The model under review builds one solid part; all positions refer to its coordinate system, in mm. A direction names the side the tool comes from. Coordinates: 2 decimals unless noted, no trailing zeros. Order: outer loops, then holes, each group sorted by start corner. A loop starts at its lowest first (then second) coordinate and runs counter-clockwise, first axis right, second up. Notation, with made-up numbers: (-12.5, 24) -> (10.5, 24) arc R10 cw to (10.5, 41) -> close; hole circle Ø8 at (-28.5, 64.25). An arc over 180 degrees is marked (long way). Use one line per item in the form item = value.
from build123d import *

# Parameters (mm, degrees)
SKETCH_1_W           = 96.5
SKETCH_1_H           = 35
EXTRUDE_1_DEPTH      = 5.2
CUT_EXTRUDE_6_DEPTH  = 1.6
CUT_EXTRUDE_7_DEPTH  = 2.6
CUT_EXTRUDE_15_DEPTH = 5
SKETCH_7_W           = 8
SKETCH_7_H           = 17
CUT_EXTRUDE_16_DEPTH = 103.736994311
SKETCH_8_W           = 18.1
SKETCH_8_H           = 16.1
CUT_EXTRUDE_17_DEPTH = 1.66
CUT_EXTRUDE_18_REACH = 104.712
SKETCH_9_W           = 15.2
SKETCH_9_H           = 16.1
CHAMFER_1_SIZE       = 0.6
SKETCH_10_W          = 12.5
SKETCH_10_H          = 12.7
CUT_EXTRUDE_19_DEPTH = 1.66
CHAMFER_2_SIZE       = 0.8
CUT_EXTRUDE_20_DEPTH = 103.782732013
CHAMFER_4_SIZE       = 1
SKETCH_14_W          = 54.3
SKETCH_14_H          = 2
EXTRUDE_2_DEPTH      = 5.2
CHAMFER_5_SIZE       = 1
CUT_EXTRUDE_21_DEPTH = 1.66
CHAMFER_3_SIZE       = 1.5
CHAMFER_6_SIZE       = 1.6
SKETCH_16_W          = 2.1
SKETCH_16_H          = 6
CUT_EXTRUDE_22_DEPTH = 104.480867797
CUT_EXTRUDE_24_DEPTH = 104.480867797
CHAMFER_11_SIZE      = 2
CHAMFER_10_SIZE      = 0.4
CUT_EXTRUDE_START    = -4.2
SKETCH_21_W          = 6.7
SKETCH_21_H          = 9.8
CUT_EXTRUDE_26_DEPTH = 4.2
CHAMFER_9_SIZE       = 1.7
SKETCH_22_W          = 16
SKETCH_22_H          = 4
CUT_EXTRUDE_27_DEPTH = 4.2
CHAMFER_12_SIZE      = 2
SKETCH_24_R          = 1.5
CUT_EXTRUDE_28_DEPTH = 104.480867797
SKETCH_25_R          = 0.85
CUT_EXTRUDE_29_DEPTH = 3
SKETCH_26_R          = 0.85
CUT_EXTRUDE_30_DEPTH = 4
SKETCH_27_W          = 20
SKETCH_27_H          = 16.1
CUT_EXTRUDE_31_DEPTH = 104.480867797
SKETCH_28_W          = 10
SKETCH_28_H          = 1.4
EXTRUDE_3_DEPTH      = 4
CHAMFER_13_SIZE      = 2
CHAMFER_14_SIZE      = 2


# Some blends are built 0.0001 mm under size
with BuildPart() as part:
    # 草图1 → 凸台-拉伸1 (new body)
    with BuildSketch(Plane(origin=(0, 0, 0), x_dir=(1, 0, 0), z_dir=(0, 1, 0))):
        with Locations((48.25, 17.5)):
            Rectangle(SKETCH_1_W, SKETCH_1_H)
    extrude(amount=EXTRUDE_1_DEPTH)

    # 草图4 → 切除-拉伸6 (cut)
    with BuildSketch(Plane(origin=(0, 5.2, 0), x_dir=(1, 0, 0), z_dir=(0, 1, 0))):
        Polygon((1.8, 6.4), (49.9, 6.4), (49.9, 9.8), (57.9, 9.8), (57.9, 28.6), (49.9, 28.6), (49.9, 32), (1.8, 32), align=None)
    extrude(amount=-CUT_EXTRUDE_6_DEPTH, mode=Mode.SUBTRACT)

    # 草图5 → 切除-拉伸7 (cut)
    with BuildSketch(Plane(origin=(0, 3.6, 0), x_dir=(1, 0, 0), z_dir=(0, 1, 0))):
        Polygon((49.9, 9), (1.8, 9), (1.8, 32), (9.9, 32), (9.9, 29.4), (16.9, 29.4), (16.9, 24), (26.9, 24), (26.9, 32), (49.9, 32), (49.9, 28.6), (57.9, 28.6), (57.9, 9.8), (49.9, 9.8), align=None)
    extrude(amount=-CUT_EXTRUDE_7_DEPTH, mode=Mode.SUBTRACT)

    # 草图6 → 切除-拉伸15 (cut, symmetric)
    with BuildSketch(Plane(origin=(0, 1, 0), x_dir=(1, 0, 0), z_dir=(0, 1, 0))):
        Polygon((3.8, 32), (8.8, 32), (8.8, 9), (1.8, 9), (1.8, 21.5), (1, 21.5), (1, 32), align=None)
    extrude(amount=CUT_EXTRUDE_15_DEPTH, both=True, mode=Mode.SUBTRACT)

    # 草图7 → 切除-拉伸16 (cut, through all)
    with BuildSketch(Plane(origin=(0, 1, 0), x_dir=(1, 0, 0), z_dir=(0, 1, 0))):
        with Locations((43.879, 19.2)):
            Rectangle(SKETCH_7_W, SKETCH_7_H)
    extrude(amount=-CUT_EXTRUDE_16_DEPTH, mode=Mode.SUBTRACT)

    # 草图8 → 切除-拉伸17 (cut)
    with BuildSketch(Plane(origin=(0, 5.2, 0), x_dir=(1, 0, 0), z_dir=(0, 1, 0))):
        with Locations((79.45, 14.45)):
            Rectangle(SKETCH_8_W, SKETCH_8_H)
    extrude(amount=-CUT_EXTRUDE_17_DEPTH, mode=Mode.SUBTRACT)

    # 草图9 → 切除-拉伸18 (cut, up to next)
    with BuildSketch(Plane(origin=(0, 3.54, 0), x_dir=(1, 0, 0), z_dir=(0, 1, 0)), mode=Mode.PRIVATE) as cut_extrude_18_sk1:
        with Locations((79.2, 14.45)):
            Rectangle(SKETCH_9_W, SKETCH_9_H)
    cut_extrude_18_tool1 = extrude(cut_extrude_18_sk1.sketch, amount=-CUT_EXTRUDE_18_REACH, mode=Mode.PRIVATE) & part.part
    add(cut_extrude_18_tool1.solids().sort_by_distance((79.2, 3.54, -14.45))[0], mode=Mode.SUBTRACT)

    # 倒角1
    chamfer_1_edges = [part.edges().sort_by_distance(p)[0] for p in [
        (47.879, 1, -19.2),
    ]]
    chamfer(chamfer_1_edges, length=CHAMFER_1_SIZE)

    # 草图10 → 切除-拉伸19 (cut)
    with BuildSketch(Plane(origin=(0, 5.2, 0), x_dir=(1, 0, 0), z_dir=(0, 1, 0))):
        with Locations((64.15, 16.15)):
            Rectangle(SKETCH_10_W, SKETCH_10_H)
    extrude(amount=-CUT_EXTRUDE_19_DEPTH, mode=Mode.SUBTRACT)

    # 倒角2
    chamfer_2_edges = [part.edges().sort_by_distance(p)[0] for p in [
        (49.9, 3.1, -28.6),
        (49.9, 3.1, -9.8),
    ]]
    chamfer(chamfer_2_edges, length=CHAMFER_2_SIZE)

    # 草图12 → 切除-拉伸20 (cut, through all)
    with BuildSketch(Plane(origin=(0, 5.2, 0), x_dir=(1, 0, 0), z_dir=(0, 1, 0))):
        Polygon((96.5, 35), (77.5, 35), (77.5, 24), (90.5, 24), (90.5, 16), (96.5, 16), align=None)
    extrude(amount=-CUT_EXTRUDE_20_DEPTH, mode=Mode.SUBTRACT)

    # 倒角4
    chamfer_4_edges = [part.edges().sort_by_distance(p)[0] for p in [
        (96.5, 2.6, -16),
    ]]
    chamfer(chamfer_4_edges, length=CHAMFER_4_SIZE)

    # 草图14 → 凸台-拉伸2 (add)
    with BuildSketch(Plane(origin=(0, 5.2, 0), x_dir=(1, 0, 0), z_dir=(0, 1, 0))):
        with Locations((48.25, 36)):
            Rectangle(SKETCH_14_W, SKETCH_14_H)
    extrude(amount=-EXTRUDE_2_DEPTH)

    # 倒角5
    chamfer_5_edges = [part.edges().sort_by_distance(p)[0] for p in [
        (21.1, 2.6, -37),
        (75.4, 2.6, -37),
    ]]
    chamfer(chamfer_5_edges, length=CHAMFER_5_SIZE)

    # 草图15 → 切除-拉伸21 (cut)
    with BuildSketch(Plane(origin=(0, 5.2, 0), x_dir=(1, 0, 0), z_dir=(0, 1, 0))):
        Polygon((77.5, 32), (57.9, 32), (57.9, 30.602488817), (57.9, 22.5), (67.9, 22.5), (67.9, 27), (77.5, 27), align=None)
    extrude(amount=-CUT_EXTRUDE_21_DEPTH, mode=Mode.SUBTRACT)

    # 倒角3
    chamfer_3_edges = [part.edges().sort_by_distance(p)[0] for p in [
        (77.5, 3.54, -29.5),
    ]]
    chamfer(chamfer_3_edges, length=CHAMFER_3_SIZE)

    # 倒角6
    chamfer_6_edges = [part.edges().sort_by_distance(p)[0] for p in [
        (1.8, 4.4, -6.4),
    ]]
    chamfer(chamfer_6_edges, length=CHAMFER_6_SIZE)

    # 草图16 → 切除-拉伸22 (cut, through all)
    with BuildSketch(Plane(origin=(0, 5.2, 0), x_dir=(1, 0, 0), z_dir=(0, 1, 0))):
        with Locations((1.05, 3)):
            Rectangle(SKETCH_16_W, SKETCH_16_H)
        with Locations((95.45, 3)):
            Rectangle(SKETCH_16_W, SKETCH_16_H)
    extrude(amount=-CUT_EXTRUDE_22_DEPTH, mode=Mode.SUBTRACT)

    # 草图19 → 切除-拉伸24 (cut, through all)
    with BuildSketch(Plane(origin=(0, 5.2, 0), x_dir=(1, 0, 0), z_dir=(0, 1, 0))):
        Polygon((15, 0), (19.2, 0), (19.2, 2), (21.2, 2), (21.2, 4.2), (13, 4.2), (13, 2), (15, 2), align=None)
        Polygon((77.3, 2), (77.3, 0), (81.5, 0), (81.5, 2), (83.5, 2), (83.5, 4.2), (75.3, 4.2), (75.3, 2), align=None)
    extrude(amount=-CUT_EXTRUDE_24_DEPTH, mode=Mode.SUBTRACT)

    # 倒角11
    chamfer_11_edges = [part.edges().sort_by_distance(p)[0] for p in [
        (83.5, 2.6, -2),
        (75.3, 2.6, -2),
        (21.2, 2.6, -2),
        (13, 2.6, -2),
    ]]
    chamfer(chamfer_11_edges, length=CHAMFER_11_SIZE - 0.0001)  # a hair under: the kernel refuses the full size

    # 倒角10
    chamfer_10_edges = [part.edges().sort_by_distance(p)[0] for p in [
        (19.2, 2.6, 0),
        (15, 2.6, 0),
        (81.5, 2.6, 0),
        (77.3, 2.6, 0),
    ]]
    chamfer(chamfer_10_edges, length=CHAMFER_10_SIZE)

    # 草图21 → 切除-拉伸26 (cut)
    with BuildSketch(Plane(origin=(0, 5.2, 0), x_dir=(1, 0, 0), z_dir=(0, 1, 0)).offset(CUT_EXTRUDE_START)):
        with Locations((56.25, 4.9)):
            Rectangle(SKETCH_21_W, SKETCH_21_H)
    extrude(amount=CUT_EXTRUDE_26_DEPTH, mode=Mode.SUBTRACT)

    # 倒角9
    chamfer_9_edges = [part.edges().sort_by_distance(p)[0] for p in [
        (57.9, 3.54, -19.2),
        (58.75, 3.54, -9.8),
    ]]
    chamfer(chamfer_9_edges, length=CHAMFER_9_SIZE - 0.0001)  # a hair under: the kernel refuses the full size

    # 草图22 → 切除-拉伸27 (cut)
    with BuildSketch(Plane(origin=(0, 5.2, 0), x_dir=(1, 0, 0), z_dir=(0, 1, 0))):
        with Locations((44.9, 2)):
            Rectangle(SKETCH_22_W, SKETCH_22_H)
    extrude(amount=-CUT_EXTRUDE_27_DEPTH, mode=Mode.SUBTRACT)

    # 倒角12
    chamfer_12_edges = [part.edges().sort_by_distance(p)[0] for p in [
        (52.9, 3.1, -4),
    ]]
    chamfer(chamfer_12_edges, length=CHAMFER_12_SIZE)

    # 草图24 → 切除-拉伸28 (cut, through all)
    with BuildSketch(Plane(origin=(0, 5.2, 0), x_dir=(1, 0, 0), z_dir=(0, 1, 0))):
        with Locations(Location((30, 3, 0), (0, 0, 270))):
            Circle(SKETCH_24_R)
        with Locations(Location((66.5, 3, 0), (0, 0, 270))):
            Circle(SKETCH_24_R)
    extrude(amount=-CUT_EXTRUDE_28_DEPTH, mode=Mode.SUBTRACT)

    # 草图25 → 切除-拉伸29 (cut)
    with BuildSketch(Plane(origin=(0, 0, -35), x_dir=(-1, 0, 0), z_dir=(0, 0, -1))):
        with Locations((-10.2, 2.6)):
            Circle(SKETCH_25_R)
    extrude(amount=-CUT_EXTRUDE_29_DEPTH, mode=Mode.SUBTRACT)

    # 草图26 → 切除-拉伸30 (cut)
    with BuildSketch(Plane.XY):
        with Locations((86.25, 3)):
            Circle(SKETCH_26_R)
    extrude(amount=-CUT_EXTRUDE_30_DEPTH, mode=Mode.SUBTRACT)

    # 草图27 → 切除-拉伸31 (cut, through all)
    with BuildSketch(Plane(origin=(0, 5.2, 0), x_dir=(1, 0, 0), z_dir=(0, 1, 0))):
        with Locations((78.5, 14.45)):
            Rectangle(SKETCH_27_W, SKETCH_27_H)
    extrude(amount=-CUT_EXTRUDE_31_DEPTH, mode=Mode.SUBTRACT)

    # 草图28 → 凸台-拉伸3 (add)
    with BuildSketch(Plane.XZ):
        with Locations((81.5, -7.1)):
            Rectangle(SKETCH_28_W, SKETCH_28_H)
        with Locations((81.5, -21.8)):
            Rectangle(SKETCH_28_W, SKETCH_28_H)
    extrude(amount=-EXTRUDE_3_DEPTH)

    # 倒角13
    chamfer_13_edges = [part.edges().sort_by_distance(p)[0] for p in [
        (68.5, 4.37, -9.8),
    ]]
    chamfer(chamfer_13_edges, length=CHAMFER_13_SIZE)

    # 倒角14
    # the kernel refuses this chamfer: 2 mm, written as the material it takes off along each edge
    with BuildSketch(Plane(origin=(68.5, 3.54, -22.5), x_dir=(-0.9996219169112968, 0.027495876610586414, 0), z_dir=(0, 0, 1))) as chamfer_14_piece_1_section:
        Polygon((CHAMFER_14_SIZE * 0.999621916911, CHAMFER_14_SIZE * 0.0274958766106), (-CHAMFER_14_SIZE * 0.0274958766106, CHAMFER_14_SIZE * 0.999621916911), (0, 0), align=None)
    chamfer_14_piece_1 = extrude(amount=19.843365976, mode=Mode.PRIVATE)
    chamfer_14_piece_1 = split(chamfer_14_piece_1, bisect_by=Plane(origin=(63.791666667, 3.073333333, -12.508333333), z_dir=(0.7071067811865476, 0, -0.7071067811865476)), keep=Keep.TOP, mode=Mode.PRIVATE)
    add(chamfer_14_piece_1, mode=Mode.SUBTRACT)


solid = part.part
Item 1: We need section B-B (z = -31). Write out the cut boundary in (x, y).
Results found:
outline = (0, 0) -> (1, 0) -> (1, 5.2) -> (0, 5.2) -> close; (8.8, 0) -> (77.5, 0) -> (77.5, 2.04) -> (76, 3.54) -> (57.9, 3.54) -> (57.9, 5.2) -> (49.9, 5.2) -> (49.9, 1) -> (26.9, 1) -> (26.9, 3.6) -> (9.9, 3.6) -> (9.9, 1) -> (8.8, 1) -> close
Item 2: We need section C-C (z = -3). Write out the cut boundary in (x, y), plus the area to 3 significant figures.
Results found:
outline = (2.1, 0) -> (14, 0) -> (14, 5.2) -> (2.1, 5.2) -> close; (20.2, 0) -> (28.5, 0) -> (28.5, 5.2) -> (20.2, 5.2) -> close; (31.5, 0) -> (65, 0) -> (65, 5.2) -> (59.6, 5.2) -> (59.6, 1) -> (36.9, 1) -> (36.9, 5.2) -> (31.5, 5.2) -> close; (68, 0) -> (76.3, 0) -> (76.3, 5.2) -> (68, 5.2) -> close; (82.5, 0) -> (94.4, 0) -> (94.4, 5.2) -> (82.5, 5.2) -> close; hole circle Ø1.7 at (86.25, 3)
area = 287 mm²
Item 3: Tool access review of faces 4 (the face through (10, 1, -35)), 5 (the face through (26, 3.6, -8)), 6 (the face through (1, 3, -27)), 7 (the face through (36.9, 3, -2)): name each direction out of +Z, -Z, +X, -X, +Y, -Y from which nothing blocks a thin tool from reaching the whole face with its end or side.
Results found:
face_4 = -Z, -X, +Y, -Y
face_5 = +Y
face_6 = +Y, -Y
face_7 = +Z, +Y
Item 4: Draft analysis for pull direction Y (two halves, no side actions). For faces 1 (the face through (87.035, 2.674, -1.972)), 2 (the face through (26.9, 2, -28)), 3 (the face through (67.49, 2.55, -15.25)), state which applies: released by +Y, released by -Y, zero draft, split by the parting line, or undercut.
Results found:
face_1 = undercut
face_2 = zero draft
face_3 = released by +Y
Item 5: We need section D-D (x = 30). Write out the cut boundary in (y, z).
Results found:
outline = (0, -37) -> (5.2, -37) -> (5.2, -32) -> (1, -32) -> (1, -9) -> (3.6, -9) -> (3.6, -6.4) -> (5.2, -6.4) -> (5.2, -4.5) -> (0, -4.5) -> close; (0, -1.5) -> (5.2, -1.5) -> (5.2, 0) -> (0, 0) -> close
Item 6: We need section A-A (x = 47). Write out the cut boundary in (y, z).
Results found:
outline = (0, -37) -> (5.2, -37) -> (5.2, -32) -> (1, -32) -> (1, -27.7) -> (0, -27.7) -> close; (0, -10.7) -> (1, -10.7) -> (1, -9) -> (3.6, -9) -> (3.6, -6.4) -> (5.2, -6.4) -> (5.2, -4) -> (1, -4) -> (1, 0) -> (0, 0) -> close
Item 7: To check wall thickness, follow L1, parallel to X at y = 1.75, z = -28.5; L2, parallel to X at y = 0.35, z = -24.5; L3, parallel to Z at x = 87.5, y = 3.4. State the ranges of each line that lie inside material, in increasing order. Write a range as from..to.
Results found:
L1 = 0..1, 16.9..26.9, 57.9..77.5
L2 = 0..1, 8.8..39.88, 47.88..77.5
L3 = -24..-22.5, -6.4..0
Item 8: Clearance check with flat-ended pins moving along their axes: pin 1 (0.5 mm diameter, centred on y = 3.5, z = -1, fed in from -X); pin 2 (2.5 mm diameter, centred on x = 1.5, y = 3, fed in from +Z); pin 3 (1.3 mm diameter, centred on x = 56, y = 4, fed in from +Z); pin 4 (6 mm diameter, centred on x = 50.5, z = -20.5, fed in from +Y). State where each tip first meets the part, or that it passes through.
Results found:
pin_1 = 2.1
pin_2 = 0
pin_3 = -28.6
pin_4 = 1
